from build123d import *

# Parameters (mm, degrees)
DOME1_FACE_RADIUS   = 2
DOME1_HEIGHT        = 2
SKETCH2_R           = 0.5
CUT_EXTRUDE1_DEPTH  = 4
SKETCH3_R           = 0.5
SKETCH3_R_2         = 0.375
EXTRUDE_THIN1_DEPTH = 50
SKETCH4_R           = 3.5
CUT_EXTRUDE2_DEPTH  = 5
SKETCH5_R           = 5
CUT_EXTRUDE3_DEPTH  = 5


with BuildPart() as part:
    # Sketch1 → Revolve1 (revolve)
    with BuildSketch(Plane.XY):
        with BuildLine():
            Line((0, 0), (0, 2))
            Line((0, 2), (-7.3, 2.899560699))
            Line((-7.3, 2.899560699), (-7.3, 4))
            ThreePointArc((-7.3, 4), (-7.8, 4.5), (-8.3, 4))
            Line((-8.3, 4), (-8.3, 3.022788192))
            Line((-8.3, 3.022788192), (-9.3, 3.146015685))
            Line((-9.3, 3.146015685), (-9.3, 4.2))
            ThreePointArc((-9.3, 4.2), (-9.8, 4.7), (-10.3, 4.2))
            Line((-10.3, 4.2), (-10.3, 3.269243178))
            Line((-10.3, 3.269243178), (-13.5, 3.663571155))
            Line((-13.5, 3.663571155), (-13.5, 5))
            Line((-13.5, 5), (-14, 5))
            Line((-14, 5), (-14, 2.969511976))
            Line((-14, 2.969511976), (-1, 1.367554567))
            Line((-1, 1.367554567), (-1, 0))
            Line((-1, 0), (0, 0))
        make_face()
    revolve(axis=Axis((0, 0, 0), (-1, 0, 0)))

    # Dome1: a dome of height H over a round flat face of radius A is a cap of a sphere of radius (A * A + H * H) / (2 * H)
    dome1_r = (DOME1_FACE_RADIUS * DOME1_FACE_RADIUS + DOME1_HEIGHT * DOME1_HEIGHT) / (2 * DOME1_HEIGHT)
    dome1_base = Plane((0, 0, 0), z_dir=(1, 0, 0))
    with Locations(dome1_base.offset(DOME1_HEIGHT - dome1_r)):
        dome1_ball = Sphere(dome1_r, mode=Mode.PRIVATE)
    add(split(dome1_ball, bisect_by=dome1_base, keep=Keep.TOP, mode=Mode.PRIVATE))

    # Sketch2 → Cut-Extrude1 (cut)
    with BuildSketch(Plane.ZY.offset(1)):
        Circle(SKETCH2_R)
    extrude(amount=-CUT_EXTRUDE1_DEPTH, mode=Mode.SUBTRACT)

    # Sketch3 → Extrude-Thin1 (add)
    with BuildSketch(Plane.ZY.offset(1)):
        Circle(SKETCH3_R)
        Circle(SKETCH3_R_2, mode=Mode.SUBTRACT)
    extrude(amount=-EXTRUDE_THIN1_DEPTH)

    # Sketch4 → Cut-Extrude2 (cut, symmetric)
    with BuildSketch(Plane.XY):
        with Locations((49, 3.5)):
            Circle(SKETCH4_R)
    extrude(amount=CUT_EXTRUDE2_DEPTH, both=True, mode=Mode.SUBTRACT)

    # Sketch5 → Cut-Extrude3 (cut, symmetric)
    with BuildSketch(Plane.XY):
        with Locations((51, 4.082575695)):
            Circle(SKETCH5_R)
    extrude(amount=CUT_EXTRUDE3_DEPTH, both=True, mode=Mode.SUBTRACT)


solid = part.part
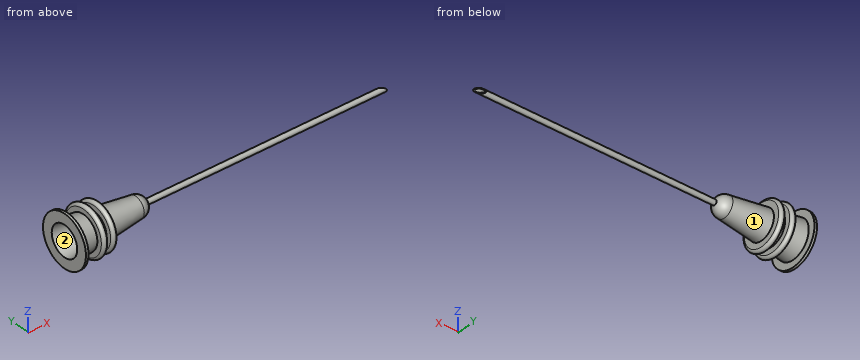
CAD build for the part. Positions are in the model's coordinates, mm. Face numbers are marked on the shaded views. Round coordinates to 2 decimals unless told otherwise and drop trailing zeros. Write each loop counter-clockwise with the first axis right and the second up, starting at its lowest first coordinate (ties: lowest second). Pieces come first, ordered by that corner, then holes.
(1) Drop flat-ended pins along their axis: P1, Ø4, axis at y = 1, z = 2, coming from the +X side; P2, Ø1, axis at x = 9, z = 0.5, coming from the +Y side; P3, Ø3, axis at y = 2.5, z = -0.5, coming from the +X side. Give the stop position or say it passes through.
(2) Mould opens along Y. For the marked faces 1 and 2 say: pulls with the +Y half, pulls with the -Y half, needs draft (parallel to the pull), parting line crosses it, or undercut.
(3) Slice it at B-B, the plane x = -2. Write the cut outline in (y, z).
(4) Probe line 1 along X through (y, z) = (-0.5, -4); line 2 along Z through (x, y) = (-6, -1.5); line 3 along X through (y, z) = (-0.75, 1). List the from-to ranges inside material, lowest first.
(5) Slice it at A-A, the plane x = 45.5. Write the cut outline in (y, z) (3 decimals), and give its area (3 significant figures).
From the geometry:
1. P1: stops at x = 48.5
1. P2: stops at y = 0.5
1. P3: stops at x = 1.7
2. face 1: parting line crosses it
2. face 2: undercut
3. outline: circle Ø4.49 at (0, 0); hole circle Ø2.98 at (0, 0)
4. line 1: x = -14 to -13.5, -10.3 to -9.3, -8.3 to -7.3
4. line 2: z = -2.29 to -1.3, 1.3 to 2.29
4. line 3: x = -1 to 1.56
5. outline: circle Ø1 at (0, 0); hole circle Ø0.75 at (0, 0)
5. area: 0.344 mm2
